Autodesk Inventor part; units mm, degrees
ref_plane "YZ Plane" through (0, 0, 0) normal (1, 0, 0) x (0, 1, 0)
ref_plane "XZ Plane" through (0, 0, 0) normal (0, 1, 0) x (-1, 0, 0)
ref_plane "XY Plane" through (0, 0, 0) normal (0, 0, 1) x (1, 0, 0)
sketch "Sketch1" plane through (0, 0, 0) normal (1, 0, 0) x (0, 1, 0)
  line L0 (0, 0) -> (50, 0)
  line L1 (50, 0) -> (50, -200)
  line L2 (50, -200) -> (0, -200)
  line L3 (0, -200) -> (0, 0)
  dimension "d0" = 50
  dimension "d1" = 200
extrude "Extrusion1" add sketch "Sketch1" along normal blind 0.602
sketch "Sketch2" plane through (0.602, 0, 0) normal (1, 0, 0) x (0, 0, -1)
  line L0 (200, 50) -> (0, 50)
  line L1 (0, 50) -> (100, 50)
  line L2 (100, 50) -> (100, 35)
  line L3 (0, 0) -> (100, 0)
  line L4 (100, 0) -> (100, 15)
  line L5 (100, 35) -> (200, 35)
  line L6 (200, 0) -> (200, 50)
  line L7 (200, 35) -> (200, 35.602)
  line L8 (200, 35.602) -> (0, 35.602)
  line L9 (0, 50) -> (0, 0)
  line L10 (0, 35.602) -> (0, 35)
  line L11 (0, 35) -> (100, 35)
  line L12 (100, 15) -> (200, 15)
  line L13 (200, 15) -> (200, 14.398)
  line L14 (200, 14.398) -> (0, 14.398)
  line L15 (0, 14.398) -> (0, 15)
  line L16 (0, 15) -> (100, 15)
  dimension "d4" = 100
  dimension "d5" = 15
  dimension "d6" = 100
  dimension "d7" = 15
  dimension "d9" = 200
  dimension "d13" = 200
extrude "Extrusion2" add sketch "Sketch2" along normal blind 19.398 contours L6 L5 L2 L8 | L2 L11 L9 L8 | L6 L14 L4 L12 | L4 L14 L9 L16
sketch "Sketch4" plane through (0.602, 35.602, 0) normal (0, 1, 0) x (1, 0, 0)
  line L0 (-0.602, 0) -> (0, 0)
  line L1 (0, 0) -> (0, 12.5)
  line L2 (0, 5) -> (0, 0)
  line L3 (0, 12.5) -> (9.699, 12.5)
  line L4 (9.699, 12.5) -> (9.699, 100)
  line L5 (9.699, 100) -> (9.699, 187.5)
  circle A0 centre (9.699, 12.5) radius 7.75
  circle A1 centre (9.699, 100) radius 7.75
  circle A2 centre (9.699, 187.5) radius 7.75
  dimension "d33" = 12.5
  dimension "d34" = 9.699
  dimension "d39" = 15.5
  dimension "d40" = 15.5
  dimension "d41" = 15.5
  dimension "d49" = 87.5
  dimension "d50" = 87.5
extrude "Extrusion4" cut sketch "Sketch4" against normal through all
sketch "Sketch6" plane through (0.602, 15, -200) normal (0, 0, -1) x (-1, 0, 0)
  point P0 (0.602, -15)
sketch "Sketch7" plane through (0, 0, -200) normal (0, 0, -1) x (-1, 0, 0)
  point P0 (0, 0)
sketch "Sketch8" plane through (0, 0, -200) normal (0, 0, -1) x (-1, 0, 0)
  line L0 (-0.602, 50) -> (-0.602, 35.602)
  line L1 (-0.602, 50) -> (-0.602, 0)
  line L2 (-0.602, 0) -> (0, 0)
  line L3 (0, 0) -> (0, 50)
  line L4 (0, 50) -> (-0.602, 50)
extrude "Extrusion6" add sketch "Sketch8" along normal blind 50
sketch "Sketch9" plane through (0, 0, 0) normal (0, 0, 1) x (1, 0, 0)
  line L0 (0, 0) -> (0, 50)
  line L1 (0, 0) -> (0, 50)
  line L2 (0, 50) -> (0.602, 50)
  line L3 (0.602, 50) -> (0.602, 0)
  line L4 (0.602, 0) -> (0, 0)
  dimension "d53" = 0.602
extrude "Extrusion7" add sketch "Sketch9" along normal blind 50
sketch "Sketch10" plane through (0, 0, 0) normal (-1, 0, 0) x (0, 0, 1)
  line L0 (0, 0) -> (-100, 0)
  line L1 (-250, 0) -> (50, 0)
  line L2 (-100, 0) -> (-100, 25)
  line L3 (-100, 25) -> (45, 25)
  line L4 (-100, 25) -> (-245, 25)
  line L5 (45.301, 50) -> (44.699, 50)
  line L6 (44.699, 50) -> (44.699, 0)
  line L7 (44.699, 0) -> (45.301, 0)
  line L8 (45.301, 0) -> (45.301, 50)
  line L9 (45.301, 50) -> (44.699, 0) construction
  line L10 (44.699, 50) -> (45.301, 0) construction
  line L11 (-245.301, 50) -> (-244.699, 50)
  line L12 (-244.699, 50) -> (-244.699, 0)
  line L13 (-244.699, 0) -> (-245.301, 0)
  line L14 (-245.301, 0) -> (-245.301, 50)
  line L15 (-245.301, 50) -> (-244.699, 0) construction
  line L16 (-244.699, 50) -> (-245.301, 0) construction
  dimension "d56" = 100
  dimension "d57" = 25
  dimension "d58" = 145
  dimension "d59" = 145
  dimension "d60" = 0.602
  dimension "d61" = 50
  dimension "d62" = 0.602
  dimension "d63" = 50
extrude "Extrusion8" add sketch "Sketch10" along normal blind 19.398 contours L6 L5 L8 L1 | L1 L14 L11 L12
sketch "Sketch11" plane through (0, 0, 45.301) normal (0, 0, 1) x (1, 0, 0)
  line L0 (0, 0) -> (-19.398, 0)
  line L1 (-19.398, 50) -> (-19.398, 0)
  line L2 (-19.398, 0) -> (-19.398, 10)
  line L3 (-19.398, 10) -> (-9.699, 10)
  line L4 (-9.699, 10) -> (-9.699, 40)
  circle A0 centre (-9.699, 10) radius 7.75
  circle A1 centre (-9.699, 40) radius 7.75
  dimension "d71" = 10
  dimension "d72" = 30
  dimension "d73" = 15.5
  dimension "d74" = 15.5
extrude "Extrusion9" [suppressed]
sketch "Sketch12" plane through (0.602, 0, 0) normal (1, 0, 0) x (0, 0, -1)
  point P0 (0, 0)
sketch "Sketch13" plane through (0.602, 50, 50) normal (0, 1, 0) x (1, 0, 0)
  point P0 (-0.602, 50)
sketch "Sketch14" plane through (0.602, 50, 50) normal (0, 1, 0) x (1, 0, 0)
  point P0 (-0.602, 50)
sketch "Sketch15" plane through (0, 0, 0) normal (-1, 0, 0) x (0, 0, 1)
  point P0 (0, 0)
equation "\"BendRadius\" = Thickness"
equation "\"BendReliefWidth\" = Thickness"
equation "\"BendReliefDepth\" = 0.5 * Thickness"
equation "\"CornerReliefSize\" = 4 * Thickness"
equation "\"MinimumRemnant\" = 2 * Thickness"
equation "\"TransitionRadius\" = BendRadius"
equation "\"JacobiRadiusSize\" = BendRadius"
equation "\"GapSize\" = Thickness"
properties part number "claw platform" material "Steel, Galvanized"
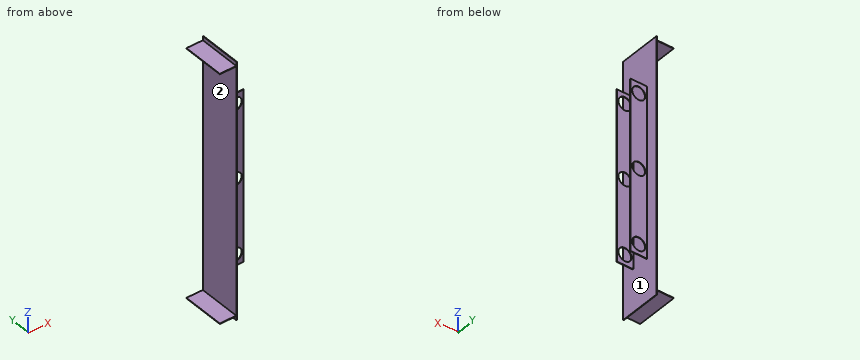
Here's how the part is built. I have some questions about the finished solid (model axes, mm). Face numbers are marked on the shaded views. Give positions to 0.01 mm unless a question says otherwise; leave off trailing zeros. Order: outer loops, then holes, each group sorted by start corner. A loop starts at its lowest first (then second) coordinate and runs counter-clockwise, first axis right, second up. Notation, with made-up numbers: (-19.5, 20.5) -> (19.5, 20.5) arc R25 ccw to (19.5, 46.5) -> close; hole circle Ø7 at (11, -29.75). An arc over 180 degrees is marked (long way). One line per item, written item: value. Start each with the question number.
1. Will these pins go through, and if not, where does the flat tip stop? pin 1 Ø18 at (x, z) = (10.301, -12.5) entering from -Y; pin 2 Ø4 at (y, z) = (19.5, -89.5) entering from -X; pin 3 Ø10 at (x, z) = (5.5, -95.5) entering from -Y; pin 4 Ø5 at (y, z) = (18, -105.5) entering from +X.
2. We'd pull the mould along Z, two halves only. Please class the marked faces 1 and 2: released by +Z, released by -Z, zero draft, split by the parting line, or undercut.
3. Imagine slicing it at C-C, the plane y = 27. List the corners of the cut face in (x, z) for me.
4. I need wall thicknesses on probe 1 along Z at (x, y) = (-2, 40); probe 2 along X at (y, z) = (35.45, -12.5); probe 3 along Y at (x, z) = (5.5, -178.5). Which ranges of each line are inside material? Lowest first, please. Write a range as from..to.
5. Imagine slicing it at A-A, the plane x = -16.5. List the corners of the cut face in (y, z) for me.
6. Imagine slicing it at D-D, the plane x = 10. Count the separate pieces of the cut face and the enclosed holes in it, plus the area to 3 significant figures.
7. Imagine slicing it at B-B, the plane z = -187.5. List the corners of the cut face in (x, y) for me, plus the area to 3 significant figures.
Values follow:
1. pin 1: stops at y = 14.4
1. pin 2: stops at x = 0
1. pin 3: stops at y = 0
1. pin 4: stops at x = 0.6
2. face 1: zero draft
2. face 2: undercut
3. outline: (-19.4, -245.3) -> (0, -245.3) -> (0, -250) -> (0.6, -250) -> (0.6, 50) -> (0, 50) -> (0, 45.3) -> (-19.4, 45.3) -> (-19.4, 44.7) -> (0, 44.7) -> (0, -244.7) -> (-19.4, -244.7) -> close
4. probe 1: z = -245.3..-244.7, 44.7..45.3
4. probe 2: x = 0..2.55, 18.05..20
4. probe 3: y = 14.4..15, 35..35.6
5. outline: (0, -245.3) -> (50, -245.3) -> (50, -244.7) -> (0, -244.7) -> close; (0, 44.7) -> (50, 44.7) -> (50, 45.3) -> (0, 45.3) -> close
6. separate pieces: 8
6. enclosed holes: 0
6. area: 185 mm2
7. outline: (0, 0) -> (0.6, 0) -> (0.6, 14.4) -> (2.55, 14.4) -> (2.55, 15) -> (0.6, 15) -> (0.6, 35) -> (2.55, 35) -> (2.55, 35.6) -> (0.6, 35.6) -> (0.6, 50) -> (0, 50) -> close; (18.05, 14.4) -> (20, 14.4) -> (20, 15) -> (18.05, 15) -> close; (18.05, 35) -> (20, 35) -> (20, 35.6) -> (18.05, 35.6) -> close
7. area: 34.8 mm2
